Read the model definition and answer for the solid it produces. Units are mm, in the model's axes. A direction names the side the tool comes from. Coordinates: 2 decimals unless noted, no trailing zeros. Order: outer loops, then holes, each group sorted by start corner. A loop starts at its lowest first (then second) coordinate and runs counter-clockwise, first axis right, second up.
```python
from build123d import *

# Parameters (mm, degrees)
CHAMFER1_SIZE      = 0.5
CUT_EXTRUDE1_REACH = 46.5
SKETCH2_R          = 1.1
SKETCH3_R          = 6.5
CUT_EXTRUDE2_DEPTH = 38


with BuildPart() as part:
    # Sketch1 → Revolve1 (revolve)
    with BuildSketch(Plane.XY):
        Polygon((-8.6, 20.75), (0, 20.75), (0, -20.75), (-6.6, -20.75), (-6.6, -27.75), (-8.6, -27.75), (-8.6, 13.75), (-14.6, 13.75), (-14.6, 16.75), (-8.6, 16.75), align=None)
    revolve(axis=Axis((0, 20.75, 0), (0, -1, 0)))

    # Chamfer1
    chamfer1_edges = [part.edges().sort_by_distance(p)[0] for p in [
        (6.6, -27.75, 0),
    ]]
    chamfer(chamfer1_edges, length=CHAMFER1_SIZE)

    # Sketch2 → Cut-Extrude1 (cut, up to next)
    with BuildSketch(Plane(origin=(0, 16.75, 0), x_dir=(1, 0, 0), z_dir=(0, 1, 0)), mode=Mode.PRIVATE) as cut_extrude1_sk1:
        with Locations((0, 12)):
            Circle(SKETCH2_R)
    cut_extrude1_tool1 = extrude(cut_extrude1_sk1.sketch, amount=-CUT_EXTRUDE1_REACH, mode=Mode.PRIVATE) & part.part
    add(cut_extrude1_tool1.solids().sort_by_distance((0, 16.75, -12))[0], mode=Mode.SUBTRACT)
    # Sketch2 → Cut-Extrude1 (cut, up to next)
    with BuildSketch(Plane(origin=(0, 16.75, 0), x_dir=(1, 0, 0), z_dir=(0, 1, 0)), mode=Mode.PRIVATE) as cut_extrude1_sk2:
        with Locations((12, 0)):
            Circle(SKETCH2_R)
    cut_extrude1_tool2 = extrude(cut_extrude1_sk2.sketch, amount=-CUT_EXTRUDE1_REACH, mode=Mode.PRIVATE) & part.part
    add(cut_extrude1_tool2.solids().sort_by_distance((12, 16.75, 0))[0], mode=Mode.SUBTRACT)
    # Sketch2 → Cut-Extrude1 (cut, up to next)
    with BuildSketch(Plane(origin=(0, 16.75, 0), x_dir=(1, 0, 0), z_dir=(0, 1, 0)), mode=Mode.PRIVATE) as cut_extrude1_sk3:
        with Locations((0, -12)):
            Circle(SKETCH2_R)
    cut_extrude1_tool3 = extrude(cut_extrude1_sk3.sketch, amount=-CUT_EXTRUDE1_REACH, mode=Mode.PRIVATE) & part.part
    add(cut_extrude1_tool3.solids().sort_by_distance((0, 16.75, 12))[0], mode=Mode.SUBTRACT)
    # Sketch2 → Cut-Extrude1 (cut, up to next)
    with BuildSketch(Plane(origin=(0, 16.75, 0), x_dir=(1, 0, 0), z_dir=(0, 1, 0)), mode=Mode.PRIVATE) as cut_extrude1_sk4:
        with Locations((-12, 0)):
            Circle(SKETCH2_R)
    cut_extrude1_tool4 = extrude(cut_extrude1_sk4.sketch, amount=-CUT_EXTRUDE1_REACH, mode=Mode.PRIVATE) & part.part
    add(cut_extrude1_tool4.solids().sort_by_distance((-12, 16.75, 0))[0], mode=Mode.SUBTRACT)

    # Sketch3 → Cut-Extrude2 (cut)
    with BuildSketch(Plane(origin=(0, 20.75, 0), x_dir=(1, 0, 0), z_dir=(0, 1, 0))):
        Circle(SKETCH3_R)
    extrude(amount=-CUT_EXTRUDE2_DEPTH, mode=Mode.SUBTRACT)


solid = part.part
```
1) Flat-ended cylindrical pins translate along their axes: pin 1 Ø4 at (x, y) = (-6, 15.5) entering from +Z; pin 2 Ø10 at (y, z) = (-8.5, -1) entering from +X; pin 3 Ø4 at (x, y) = (0, -7.5) entering from -Z. Find the tip coordinate at first contact, or state that the pin passes through.
A:
pin 1: stops at z = 14.04
pin 2: stops at x = 8.6
pin 3: stops at z = -8.6
2) A cutting plane is placed at A-A, the plane x = 0. State how many separate pieces and enclosed holes the cut face has, and give its area (3 significant figures).
A:
separate pieces: 3
enclosed holes: 0
area: 270 mm2
3) Which of the six approach directions +Z, -Z, +X, -X, +Y, -Y give full straight-line access (tool end or side, diameter ignored) to faces 4 (the cylindrical face through (8.59, -6.71, -0.38)), 5 (the cylindrical face through (-5.158, 2.016, 3.955)), 6 (the cylindrical face through (13.016, 15.271, 0.421))?
A:
face 4: -Y
face 5: +Y
face 6: +Y, -Y
4) Straight lines are drawn through the part: line 1 (Z direction, x = 0, y = 16.05); line 2 (Z direction, x = 0, y = -25). For each, find the intervals that lie inside material, in ascending order.
A:
line 1: z = -14.6 to -13.1, -10.9 to -6.5, 6.5 to 10.9, 13.1 to 14.6
line 2: z = -8.6 to -6.6, 6.6 to 8.6
5) Determine the mould class of faces 1 (the flat face through (6.3, 13.75, 6.3)), 2 (the flat face through (0, -20.75, 0)), 3 (the cylindrical face through (8.59, 18.78, -0.38)) for opening direction Z: pulls with the +Z half, pulls with the -Z half, needs draft (parallel to the pull), parting line crosses it, or undercut.
A:
face 1: needs draft
face 2: undercut
face 3: parting line crosses it
6) A cutting plane is placed at D-D, the plane y = 3.5. Determine the outline of the cut face in (x, z).
A:
outline: circle Ø17.2 at (0, 0); hole circle Ø13 at (0, 0)
7) A cutting plane is placed at C-C, the plane x = 12. Determine the outline of the cut face in (y, z), and give its area (3 significant figures).
A:
outline: (13.75, -8.32) - (16.75, -8.32) - (16.75, -1.1) - (13.75, -1.1) - close; (13.75, 1.1) - (16.75, 1.1) - (16.75, 8.32) - (13.75, 8.32) - close
area: 43.3 mm2
8) A cutting plane is placed at B-B, the plane z = 12. Determine the outline of the cut face in (x, y).
A:
outline: (-8.32, 13.75) - (-1.1, 13.75) - (-1.1, 16.75) - (-8.32, 16.75) - close; (1.1, 13.75) - (8.32, 13.75) - (8.32, 16.75) - (1.1, 16.75) - close
